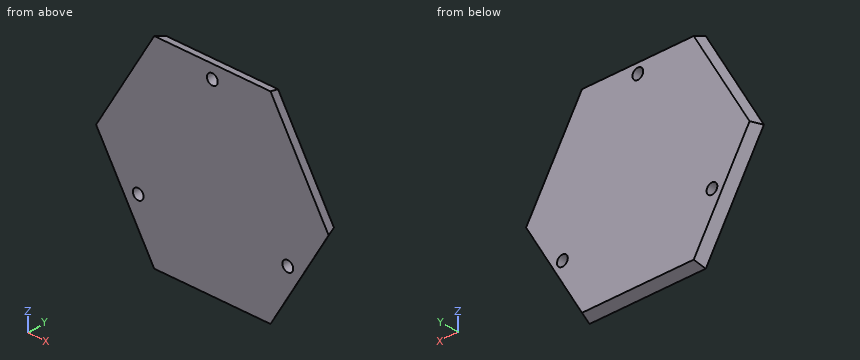
from build123d import *

# Parameters (mm, degrees)
BOSS_EXTRUDE1_DEPTH = 10
BOSS_EXTRUDE1_TAPER = -20
SKETCH1_4_R         = 5
CUT_EXTRUDE1_DEPTH  = 10


with BuildPart() as part:
    # Sketch1 → Boss-Extrude1 (new body)
    with BuildSketch(Plane(origin=(0, 0, 0), x_dir=(1, 0, 0), z_dir=(0, 1, 0))):
        Polygon((103.923048454, 0), (51.961524227, 90), (-51.961524227, 90), (-103.923048454, 0), (-51.961524227, -90), (51.961524227, -90), align=None)
    extrude(amount=-BOSS_EXTRUDE1_DEPTH, taper=BOSS_EXTRUDE1_TAPER)

    # Sketch1<4> → Cut-Extrude1 (cut)
    with BuildSketch(Plane(origin=(0, 0, 0), x_dir=(1, 0, 0), z_dir=(0, 1, 0))):
        with Locations((0, -81)):
            Circle(SKETCH1_4_R)
        with Locations((70.148057707, 40.5)):
            Circle(SKETCH1_4_R)
        with Locations((-68.942286341, 39.803847577)):
            Circle(SKETCH1_4_R)
    extrude(amount=-CUT_EXTRUDE1_DEPTH, mode=Mode.SUBTRACT)


solid = part.part
CAD build for the part. Positions are in the model's coordinates, mm. Give positions to 0.01 mm unless a question says otherwise; leave off trailing zeros. Write each question's results on one line, items separated by ' | '.
1. Probe L1, parallel to X at y = -4.75, z = -40.5; L2, parallel to X at y = -7.5, z = 81; L3, parallel to X at y = -4.25, z = -40.5. List the from-to ranges inside material, lowest first. Write a range as from..to.
Calculated:
L1: x = -82.54..-73.89, -63.99..65.15, 75.15..82.54 | L2: x = -60.31..-5, 5..60.31 | L3: x = -82.33..-73.89, -63.99..65.15, 75.15..82.33
2. Saw through at A-A on y = -6. Count the separate pieces of the cut face and the enclosed holes in it, and give its area (3 significant figures).
Calculated:
separate pieces: 1 | enclosed holes: 3 | area: 29,200 mm2
3. Pin check, flat tips, straight feed: pin 1 (6 mm diameter, centred on x = 0, z = 81, fed in from +Y); pin 2 (6 mm diameter, centred on x = -86.5, y = -5.5, fed in from +Z); pin 3 (1 mm diameter, centred on x = 35.5, y = -8.5, fed in from -Z); pin 4 (2 mm diameter, centred on y = -3.5, z = 9, fed in from +X). Stop position of each tip, or through.
Calculated:
pin 1: passes through | pin 2: stops at z = 39.82 | pin 3: stops at z = -93.28 | pin 4: stops at x = 100.91
